Part model, mm, in its own coordinate system. Face numbers are marked on the shaded views. A direction names the side the tool comes from. Coordinates: 2 decimals unless noted, no trailing zeros. Write each loop counter-clockwise with the first axis right and the second up, starting at its lowest first coordinate (ties: lowest second). Pieces come first, ordered by that corner, then holes. Notation, with made-up numbers: (42.25, 13) - (57.25, 13) arc R24 ccw to (57.25, 52) - close; hole circle Ø10 at (61.5, -5.75). An arc over 180 degrees is marked (long way). Use one line per item in the form item = value. Start each with the question number.
from build123d import *

# Parameters (mm, degrees)
BASE_FLANGE1_DEPTH    = 13
FILLET1_R             = 6.5
M5X0_8_TAPPED_HOLE1_D = 4.2
M5X0_8_TAPPED_HOLE2_D = 4.2


# Sheet-metal steps are written as plain solids
with BuildPart() as part:
    # Sketch1 → Base-Flange1 (new body)
    with BuildSketch(Plane.XY):
        with BuildLine():
            Line((13.25, 13.25), (-10.45, 13.25))
            ThreePointArc((-10.45, 13.25), (-12.429898987, 12.429898987), (-13.25, 10.45))
            Line((-13.25, 10.45), (-13.25, -13.25))
            Line((-13.25, -13.25), (-11.25, -13.25))
            Line((-11.25, -13.25), (-11.25, 10.45))
            ThreePointArc((-11.25, 10.45), (-11.015685425, 11.015685425), (-10.45, 11.25))
            Line((-10.45, 11.25), (13.25, 11.25))
            Line((13.25, 11.25), (13.25, 13.25))
        make_face()
    extrude(amount=BASE_FLANGE1_DEPTH)

    # Fillet1
    fillet1_edges = [part.edges().sort_by_distance(p)[0] for p in [
        (-12.25, -13.25, 0),
        (-12.25, -13.25, 13),
        (13.25, 12.25, 0),
        (13.25, 12.25, 13),
    ]]
    fillet(fillet1_edges, radius=FILLET1_R - 0.0001)  # a hair under: the kernel refuses the full size

    # M5x0.8 Tapped Hole1 (through all)
    with Locations(Plane(origin=(0, 13.25, 0), x_dir=(-1, 0, 0), z_dir=(0, 1, 0))):
        with Locations((-6.75, 6.5)):
            Hole(M5X0_8_TAPPED_HOLE1_D / 2)

    # M5x0.8 Tapped Hole2 (through all)
    with Locations(Plane.ZY.offset(13.25)):
        with Locations((6.5, -6.75)):
            Hole(M5X0_8_TAPPED_HOLE2_D / 2)


solid = part.part
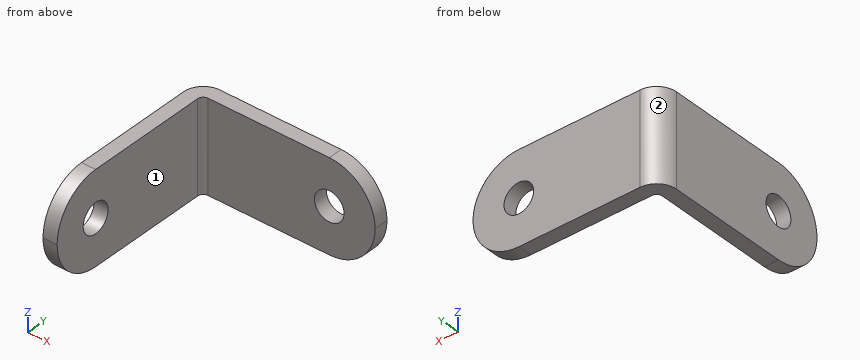
Q1. Pin check, flat tips, straight feed: P1, Ø6.5, axis at y = 3, z = 4.5, coming from the +X side; P2, Ø6, axis at x = 10, z = 6, coming from the -Y side; P3, Ø3.5, axis at x = 6.75, z = 6.5, coming from the +Y side. Stop position of each tip, or through.
Q2. Slice it at B-B (x = 5.5). List the corners of the cut face in (y, z).
Q3. Slice it at D-D (z = 4). List the corners of the cut face in (x, y), plus the area to 3 significant figures.
Q4. Which spindle directions (+Z, -Z, +X, -X, +Y, -Y) get a long thin tool onto all of the face, cutting with end or side? Do the marked faces 1 and 2. Say none if no direction does.
Q5. Slice it at C-C (z = 8). List the corners of the cut face in (x, y).
Q6. Slice it at A-A (y = -6). List the corners of the cut face in (x, z).
Q7. Drill centre lines: probe 1 along X at (y, z) = (-10.5, 6.5); probe 2 along Z at (x, y) = (6.75, 11.9); probe 3 along Y at (x, z) = (4.5, 8). Where is each one in solid material? Low to high.
Solution:
q1.P1 = -11.25
q1.P2 = 11.25
q1.P3 = through
q2.outline = (11.25, 0) - (13.25, 0) - (13.25, 4.81) - (11.25, 4.81) - close; (11.25, 8.19) - (13.25, 8.19) - (13.25, 13) - (11.25, 13) - close
q3.outline = (-13.25, -12.75) - (-11.25, -12.75) - (-11.25, 10.45) arc R0.8 cw to (-10.45, 11.25) - (12.75, 11.25) - (12.75, 13.25) - (-10.45, 13.25) arc R2.8 ccw to (-13.25, 10.45) - close
q3.area = 98.5 mm2
q4.face_1 = +Z, -Z, +X, -Y
q4.face_2 = +Z, -Z, -X, +Y
q5.outline = (-13.25, -13.07) - (-11.25, -13.07) - (-11.25, -8.22) - (-13.25, -8.22) - close; (-13.25, -5.28) - (-11.25, -5.28) - (-11.25, 10.45) arc R0.8 cw to (-10.45, 11.25) - (5.28, 11.25) - (5.28, 13.25) - (-10.45, 13.25) arc R2.8 ccw to (-13.25, 10.45) - close; (8.22, 11.25) - (13.07, 11.25) - (13.07, 13.25) - (8.22, 13.25) - close
q6.outline = (-13.25, 0) - (-11.25, 0) - (-11.25, 4.54) - (-13.25, 4.54) - close; (-13.25, 8.46) - (-11.25, 8.46) - (-11.25, 13) - (-13.25, 13) - close
q7.probe_1 = -13.25 to -11.25
q7.probe_2 = 0 to 4.4, 8.6 to 13
q7.probe_3 = 11.25 to 13.25
